Build history of the part. All positions in model axes, mm. Face numbers are marked on the shaded views. A direction names the side the tool comes from. Give positions to 0.01 mm unless a question says otherwise; leave off trailing zeros. Loops run counter-clockwise (first coordinate to the right, second up) from the corner with the lowest first, then second, coordinate; pieces in that order, holes last. Notation, with made-up numbers: M 15.25,-26 L 21.25,-26 A22 cw 21.25,0 Z; hole C -18.5,-36 d5. An arc over 180 degrees is marked long. Put each result on its own line as item: value.
```python
from build123d import *

# Parameters (mm, degrees)
F0_R = 1.875
F3_R = 1
F4_R = 0.5


with BuildPart() as f2:
    # F2: sweep along a path in F1
    with BuildLine(Plane.YZ) as f2_path:
        Line((0, 0), (-11.5, 0))
        Line((-11.5, 0), (-16.5714191409, 10.8756934444))
    # F0 (on Front) → F2 (sweep)
    with BuildSketch(Plane.XZ):
        Circle(F0_R)
    sweep(path=f2_path.line, transition=Transition.RIGHT)

    # F3
    f3_edges = [f2.edges().sort_by_distance(p)[0] for p in [
        (-1.875, 0, 0),
    ]]
    fillet(f3_edges, radius=F3_R)

    # F4
    f4_edges = [f2.edges().sort_by_distance(p)[0] for p in [
        (-1.875, -16.571419, 10.875693),
    ]]
    fillet(f4_edges, radius=F4_R)


solid = f2.part
```
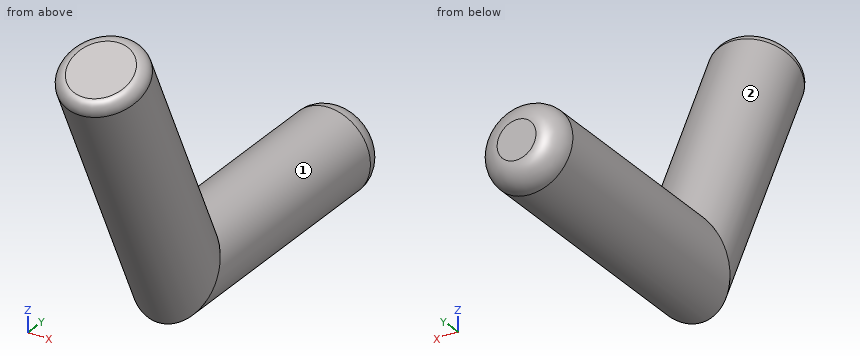
Q1. Drop flat-ended pins along their axis: pin 1 Ø1 at (x, y) = (0, -14) entering from -Z; pin 2 Ø1 at (x, y) = (0.5, -3) entering from +Z (3 decimals). Give the stop position or say it passes through.
Here are the results:
pin 1: z = -0.15
pin 2: z = 1.875
Q2. Slice it at A-A (y = -8.75). List the corners of the cut face in (x, z) (3 decimals).
Here are the results:
outline: C 0,0 d3.75
Q3. Tool access for the marked faces 1 and 2: list every direction of +Z, -Z, +X, -X, +Y, -Y with a clear straight run to the whole face (end or side of a thin tool).
Here are the results:
face 1: +Y
face 2: none
Q4. Probe line 1 (Z direction, x = 0, y = -4) (3 decimals); line 2 (Y direction, x = 1.55, z = 9.5); line 3 (Y direction, x = 0.8, z = 10). List the from-to ranges inside material, lowest first. Write a range as from..to.
Here are the results:
line 1: -1.875..1.875
line 2: -17.09..-14.77
line 3: -17.93..-14.29
